from build123d import *

# Parameters (mm, degrees)
SKETCH_1_W          = 62
SKETCH_1_H          = 10
EXTRUDE_1_DEPTH     = 15
SKETCH_2_R          = 6.5
CUT_EXTRUDE_1_DEPTH = 5
SKETCH_4_R          = 3.5
CUT_EXTRUDE_3_DEPTH = 53.440442409
SKETCH_3_W          = 13.191362224
SKETCH_3_H          = 26.166472608
CUT_EXTRUDE_2_DEPTH = 54.150729064


with BuildPart() as part:
    # 草图1 → 凸台-拉伸1 (new, symmetric)
    with BuildSketch(Plane(origin=(0, 0, 0), x_dir=(0, 0, -1), z_dir=(1, 0, 0))):
        with Locations((19, 0)):
            Rectangle(SKETCH_1_W, SKETCH_1_H)
    extrude(amount=EXTRUDE_1_DEPTH, both=True)

    # 草图2 → 切除-拉伸1 (cut)
    with BuildSketch(Plane(origin=(0, -5, 0), x_dir=(1, 0, 0), z_dir=(0, 1, 0))):
        with Locations(Location((0, 0, 0), (0, 0, 270))):
            Circle(SKETCH_2_R)
    extrude(amount=CUT_EXTRUDE_1_DEPTH, mode=Mode.SUBTRACT)

    # 草图4 → 切除-拉伸3 (cut, through all)
    with BuildSketch(Plane.XZ):
        with Locations(Location((0, 0, 0), (0, 0, 270))):
            Circle(SKETCH_4_R)
    extrude(amount=-CUT_EXTRUDE_3_DEPTH, mode=Mode.SUBTRACT)

    # 草图3 → 切除-拉伸2 (cut, through all)
    with BuildSketch(Plane(origin=(0, 5, 0), x_dir=(1, 0, 0), z_dir=(0, 1, 0))):
        with Locations((0, 30)):
            Rectangle(SKETCH_3_W, SKETCH_3_H)
    extrude(amount=-CUT_EXTRUDE_2_DEPTH, mode=Mode.SUBTRACT)


solid = part.part
Check sheet for the modelled part. Datum: model origin and axes. Units: mm. A direction names the side the tool comes from. Round coordinates to 2 decimals unless told otherwise and drop trailing zeros. Loops run counter-clockwise (first coordinate to the right, second up) from the corner with the lowest first, then second, coordinate; pieces in that order, holes last. Notation, with made-up numbers: M 70.5,-25 L 91.5,-25 A22 cw 91.5,-19 Z; hole C 46.5,8.25 d1. An arc over 180 degrees is marked long. One line per question, with ' | ' between items. Start each with the question number.
Item 1: Section check A-A (z = -22). Record the boundary of the cut face in (x, y).
Item 2: Set-up check for faces 1 (the face through (0, -5, -12)), 2 (the face through (-3, 0, 3)), 3 (the face through (0, 0, -16.917)): record each of +Z, -Z, +X, -X, +Y, -Y from which the full face is reachable in a straight line by a thin tool's end or side.
Item 3: Scan lines: probe 1 along X at (y, z) = (-2.25, -42.5); probe 2 along Z at (x, y) = (4.5, -0.25); probe 3 along X at (y, z) = (1.95, 0). Record each from-to range of solid material in increasing order.
Item 4: Release check for a two-part mould opening along Z. For faces 4 (the face through (6.596, 0, -30)), 5 (the face through (0, 5, -12)), 6 (the face through (0, 0, 12)), 7 (the face through (-3.417, 2.465, 0.759)) record: released by +Z, released by -Z, zero draft, split by the parting line, or undercut.
Item 5: Section check D-D (y = -1). Record the boundary of the cut face in (x, z).
Item 6: Section check B-B (x = 0). Record the boundary of the cut face in (y, z).
Item 7: Section check C-C (y = 3.5). Record the boundary of the cut face in (x, z).
Worked out:
1) outline: M -15,-5 L -6.6,-5 L -6.6,5 L -15,5 Z; M 6.6,-5 L 15,-5 L 15,5 L 6.6,5 Z
2) face 1: +Z, -Z, +X, -X, -Y | face 2: -Y | face 3: +Y, -Y
3) probe 1: -15 to -6.6, 6.6 to 15 | probe 2: -50 to -43.08, -16.92 to -4.69, 4.69 to 12 | probe 3: -15 to -3.5, 3.5 to 15
4) face 4: undercut | face 5: zero draft | face 6: released by +Z | face 7: undercut
5) outline: M -15,-50 L 15,-50 L 15,12 L -15,12 Z; hole M -6.6,-43.08 L 6.6,-43.08 L 6.6,-16.92 L -6.6,-16.92 Z; hole C 0,0 d13
6) outline: M -5,-50 L 5,-50 L 5,-43.08 L -5,-43.08 Z; M -5,-16.92 L 5,-16.92 L 5,-3.5 L 0,-3.5 L 0,-6.5 L -5,-6.5 Z; M -5,6.5 L 0,6.5 L 0,3.5 L 5,3.5 L 5,12 L -5,12 Z
7) outline: M -15,-50 L 15,-50 L 15,12 L -15,12 Z; hole M -6.6,-43.08 L 6.6,-43.08 L 6.6,-16.92 L -6.6,-16.92 Z; hole C 0,0 d7
